The listing builds one solid part. Answer for the finished solid, in the listing's coordinates (mm). Face numbers are marked on the shaded views. A direction names the side the tool comes from. Give positions to 0.01 mm unless a question says otherwise; leave off trailing zeros. Order: outer loops, then holes, each group sorted by start corner. A loop starts at its lowest first (then second) coordinate and runs counter-clockwise, first axis right, second up.
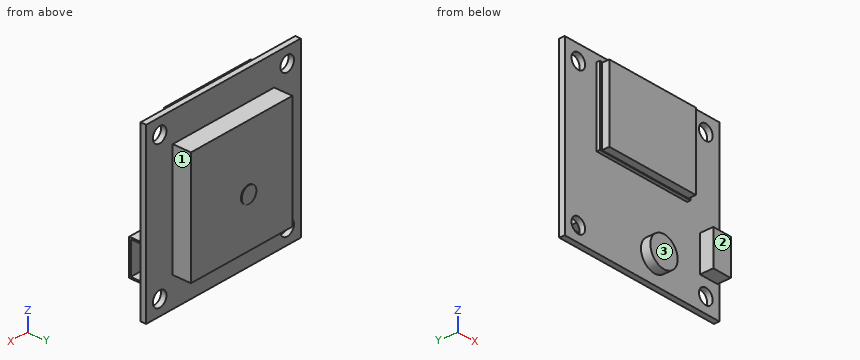
```python
from build123d import *

# Parameters (mm, degrees)
SKETCH1_W           = 38.354
SKETCH1_H           = 38.2778
BOARD_DEPTH         = 1.2319
SKETCH3_W           = 25.146
SKETCH3_H           = 25.146
GPS_DEPTH           = 4.0767
SKETCH5_W           = 21.4376
SKETCH5_H           = 16.7894
UBLOCK_CHIP_DEPTH   = 2.4257
SKETCH6_R           = 3.3782
BATTERY_DEPTH       = 2.1082
SKETCH7_W           = 4.318
SKETCH7_H           = 7.9502
CONNECTOR_DEPTH     = 2.9972
SKETCH8_W           = 7.239
SKETCH8_H           = 2.286
CUT_EXTRUDE1_DEPTH  = 3.7592
CUT_EXTRUDE2_REACH  = 56.352
SKETCH9_R           = 1.6891
SKETCH10_R          = 1.8161
BOSS_EXTRUDE6_DEPTH = 0.1778
SKETCH11_W          = 22.479
SKETCH11_H          = 17.1323
BOSS_EXTRUDE7_DEPTH = 0.762


with BuildPart() as part:
    # Sketch1 → Board (new body)
    with BuildSketch(Plane(origin=(0, 0, 0), x_dir=(1, 0, 0), z_dir=(0, 1, 0))):
        with Locations((19.177, 19.1389)):
            Rectangle(SKETCH1_W, SKETCH1_H)
    extrude(amount=BOARD_DEPTH)

    # Sketch3 → GPS (add)
    with BuildSketch(Plane(origin=(0, 1.2319, 0), x_dir=(1, 0, 0), z_dir=(0, 1, 0))):
        with Locations((19.177, 19.1389)):
            Rectangle(SKETCH3_W, SKETCH3_H)
    extrude(amount=GPS_DEPTH)

    # Sketch5 → uBlock chip (add)
    with BuildSketch(Plane.XZ):
        with Locations((19.1008, -10.2108)):
            Rectangle(SKETCH5_W, SKETCH5_H)
    extrude(amount=UBLOCK_CHIP_DEPTH)

    # Sketch6 → Battery (add)
    with BuildSketch(Plane(origin=(0, 0, 0), x_dir=(-1, 0, 0), z_dir=(0, -1, 0))):
        with Locations(Location((-22.2758, 32.6263, 0), (0, 0, 90))):
            Circle(SKETCH6_R)
    extrude(amount=BATTERY_DEPTH)

    # Sketch7 → Connector (add)
    with BuildSketch(Plane(origin=(0, 0, 0), x_dir=(-1, 0, 0), z_dir=(0, -1, 0))):
        with Locations((-35.687, 27.3304)):
            Rectangle(SKETCH7_W, SKETCH7_H)
    extrude(amount=CONNECTOR_DEPTH)

    # Sketch8 → Cut-Extrude1 (cut)
    with BuildSketch(Plane(origin=(37.846, 0, 0), x_dir=(0, 0, -1), z_dir=(1, 0, 0))):
        with Locations((27.3304, -1.4986)):
            Rectangle(SKETCH8_W, SKETCH8_H)
    extrude(amount=-CUT_EXTRUDE1_DEPTH, mode=Mode.SUBTRACT)

    # Sketch9 → Cut-Extrude2 (cut, up to next)
    with BuildSketch(Plane(origin=(0, 1.2319, 0), x_dir=(1, 0, 0), z_dir=(0, 1, 0)), mode=Mode.PRIVATE) as cut_extrude2_sk1:
        with Locations(Location((34.9885, 3.3655, 0), (0, 0, 270))):
            Circle(SKETCH9_R)
    cut_extrude2_tool1 = extrude(cut_extrude2_sk1.sketch, amount=-CUT_EXTRUDE2_REACH, mode=Mode.PRIVATE) & part.part
    # Sketch9 → Cut-Extrude2 (cut, up to next)
    with BuildSketch(Plane(origin=(0, 1.2319, 0), x_dir=(1, 0, 0), z_dir=(0, 1, 0)), mode=Mode.PRIVATE) as cut_extrude2_sk2:
        with Locations(Location((3.3655, 3.3655, 0), (0, 0, 270))):
            Circle(SKETCH9_R)
    cut_extrude2_tool2 = extrude(cut_extrude2_sk2.sketch, amount=-CUT_EXTRUDE2_REACH, mode=Mode.PRIVATE) & part.part
    # Sketch9 → Cut-Extrude2 (cut, up to next)
    with BuildSketch(Plane(origin=(0, 1.2319, 0), x_dir=(1, 0, 0), z_dir=(0, 1, 0)), mode=Mode.PRIVATE) as cut_extrude2_sk3:
        with Locations(Location((3.3655, 34.9123, 0), (0, 0, 270))):
            Circle(SKETCH9_R)
    cut_extrude2_tool3 = extrude(cut_extrude2_sk3.sketch, amount=-CUT_EXTRUDE2_REACH, mode=Mode.PRIVATE) & part.part
    # Sketch9 → Cut-Extrude2 (cut, up to next)
    with BuildSketch(Plane(origin=(0, 1.2319, 0), x_dir=(1, 0, 0), z_dir=(0, 1, 0)), mode=Mode.PRIVATE) as cut_extrude2_sk4:
        with Locations(Location((34.9885, 34.9123, 0), (0, 0, 270))):
            Circle(SKETCH9_R)
    cut_extrude2_tool4 = extrude(cut_extrude2_sk4.sketch, amount=-CUT_EXTRUDE2_REACH, mode=Mode.PRIVATE) & part.part
    add(cut_extrude2_tool1.solids().sort_by_distance((34.9885, 1.2319, -3.3655))[0], mode=Mode.SUBTRACT)
    add(cut_extrude2_tool2.solids().sort_by_distance((3.3655, 1.2319, -3.3655))[0], mode=Mode.SUBTRACT)
    add(cut_extrude2_tool3.solids().sort_by_distance((3.3655, 1.2319, -34.9123))[0], mode=Mode.SUBTRACT)
    add(cut_extrude2_tool4.solids().sort_by_distance((34.9885, 1.2319, -34.9123))[0], mode=Mode.SUBTRACT)

    # Sketch10 → Boss-Extrude6 (add)
    with BuildSketch(Plane(origin=(0, 5.3086, 0), x_dir=(1, 0, 0), z_dir=(0, 1, 0))):
        with Locations(Location((17.5387, 20.7518, 0), (0, 0, 90))):
            Circle(SKETCH10_R)
    extrude(amount=BOSS_EXTRUDE6_DEPTH)

    # Sketch11 → Boss-Extrude7 (add)
    with BuildSketch(Plane.XZ):
        with Locations((19.1008, -10.2108)):
            Rectangle(SKETCH11_W, SKETCH11_H)
    extrude(amount=BOSS_EXTRUDE7_DEPTH)


solid = part.part
```
1) Find section C-C (z = -3). Write down the section's boundary in (x, y), then the cut area to 3 significant figures.
Geometry says:
outline: (0, 0) - (1.72, 0) - (1.72, 1.23) - (0, 1.23) - close; (5.01, 0) - (7.86, 0) - (7.86, -0.76) - (8.38, -0.76) - (8.38, -2.43) - (29.82, -2.43) - (29.82, -0.76) - (30.34, -0.76) - (30.34, 0) - (33.34, 0) - (33.34, 1.23) - (5.01, 1.23) - close; (36.64, 0) - (38.35, 0) - (38.35, 1.23) - (36.64, 1.23) - close
area: 91.9 mm2
2) Straight lines are drawn through the part: probe 1 along Z at (x, y) = (35, -1.5); probe 2 along Z at (x, y) = (34, 1); probe 3 along Z at (x, y) = (34.5, 0.25). For each, find the intervals that lie inside material, in ascending order.
Geometry says:
probe 1: z = -31.31 to -30.95, -23.71 to -23.36
probe 2: z = -38.28 to -36.28, -33.54 to -4.74, -2 to 0
probe 3: z = -38.28 to -36.53, -33.3 to -4.98, -1.75 to 0
3) Find section D-D (y = 0.75). Write down the section's boundary in (x, z).
Geometry says:
outline: (0, -38.28) - (38.35, -38.28) - (38.35, 0) - (0, 0) - close; hole circle Ø3.38 at (3.37, -34.91); hole circle Ø3.38 at (3.37, -3.37); hole circle Ø3.38 at (34.99, -34.91); hole circle Ø3.38 at (34.99, -3.37)
4) A tool of negligible diameter and unlimited length cuts with its end or side. For the marked faces 1, 2 and 3, from which of +Z, -Z, +X, -X, +Y, -Y can it reach the whole face along a straight path? Write none if from no direction.
Geometry says:
face 1: +Z, -Z, +X, +Y
face 2: +Z, -Z, +X, -X, -Y
face 3: -Z, -X, -Y
5) Find section B-B (z = -11.5). Write down the section's boundary in (x, y).
Geometry says:
outline: (0, 0) - (7.86, 0) - (7.86, -0.76) - (8.38, -0.76) - (8.38, -2.43) - (29.82, -2.43) - (29.82, -0.76) - (30.34, -0.76) - (30.34, 0) - (38.35, 0) - (38.35, 1.23) - (31.75, 1.23) - (31.75, 5.31) - (6.6, 5.31) - (6.6, 1.23) - (0, 1.23) - close
6) Given P1, Ø3, axis at x = 20, y = -2, coming from the -Z side; P2, Ø0.8, axis at x = 24, y = -1.5, coming from the +Z side; P3, Ø4.5, axis at x = 34.99, z = -3.37, coming from the -Y side; P4, Ø3, axis at x = 3.37, z = -3.37, coming from the +Y side, each flat-ended and moving along its own axis, determine where each tip first touches the part or whether it passes through.
Geometry says:
P1: stops at z = -35.91
P2: stops at z = -1.82
P3: stops at y = 0
P4: passes through
7) Find section A-A (x = 13). Write down the section's boundary in (y, z), then the cut area to 3 significant figures.
Geometry says:
outline: (-2.43, -18.61) - (-0.76, -18.61) - (-0.76, -18.78) - (0, -18.78) - (0, -38.28) - (1.23, -38.28) - (1.23, -31.71) - (5.31, -31.71) - (5.31, -6.57) - (1.23, -6.57) - (1.23, 0) - (0, 0) - (0, -1.64) - (-0.76, -1.64) - (-0.76, -1.82) - (-2.43, -1.82) - close
area: 191 mm2
